Input: part model. Units: mm. Frame: model coordinates. A direction names the side the tool comes from. Coordinates: 2 decimals unless noted, no trailing zeros. Write each loop counter-clockwise with the first axis right and the second up, starting at its lowest first coordinate (ties: lowest second). Pieces come first, ordered by that corner, then holes. Notation, with made-up numbers: (44, -21) - (74, -21) arc R25 ccw to (74, -5) - close; hole circle Ø6 at (-23.5, 16.5). An arc over 180 degrees is marked (long way). Use a Markdown table: item, result. Add a question column.
Q1. Pin query (flat end, axial travel): P1, Ø1.9, axis at x = 15.5, z = 15.5, coming from the +Y side; P2, Ø2.5, axis at x = 86, z = 1, coming from the -Y side; P3, Ø7, axis at x = 2.5, z = 3, coming from the +Y side; P4, Ø2, axis at x = 9.5, z = 16.5, coming from the +Y side. Return the tip coordinate at first contact, or that it passes through.
Q2. Section query B-B (x = -85). Return the cut outline in (y, z) (3 decimals), then the cut area to 3 significant figures.
Q3. Set-up query: faces 1 (the face through (88.72, 3.94, -1.54)), 2 (the face through (93.5, 5.07, -19.72)), 3 (the face through (5.19, 6.77, 9.98)). Return all of +Z, -Z, +X, -X, +Y, -Y with unobstructed straight access to the full face (end or side cutting, diameter ignored); none if empty.
Q4. Section query A-A (x = -33.25). Return the cut outline in (y, z).
Q5. Section query C-C (z = -8). Return the cut outline in (x, y).
Q6. Section query D-D (x = 75). Return the cut outline in (y, z).
Q7. Material intervals for probe 1 along Z at (x, y) = (15.5, 4); probe 2 along Z at (x, y) = (-33.25, 4); probe 3 along X at (y, z) = (4, 15.5), sorted ascending. Write a range as from..to.
Q8. Mould query, pull axis X, two halves, no side actions, for faces 4 (the face through (-1.08, 2.79, 4.88)), 5 (the face through (-59, 10, 0)), 6 (the face through (95, 5, 0)). Classes: released by +X, released by -X, zero draft, split by the parting line, or undercut.
from build123d import *

# Parameters (mm, degrees)
SKETCH_1_W          = 190
SKETCH_1_H          = 42.3
EXTRUDE_1_DEPTH     = 10
SKETCH_2_W          = 42.5
SKETCH_2_H          = 49.677136544
CUT_EXTRUDE_1_DEPTH = 2
SKETCH_3_R          = 1.6
SKETCH_3_R_2        = 11.25
CUT_EXTRUDE_2_DEPTH = 2.5
SKETCH_4_R          = 5
CUT_EXTRUDE_3_DEPTH = 6.5
SKETCH_5_R          = 4.025
CUT_EXTRUDE_4_DEPTH = 8
SKETCH_6_R          = 1.6
CUT_EXTRUDE_5_DEPTH = 3
SKETCH_7_R          = 1.6
CUT_EXTRUDE_6_DEPTH = 3
FILLET_1_R          = 5
SKETCH_8_R          = 1.6
CUT_EXTRUDE_7_DEPTH = 9
CUT_EXTRUDE_8_REACH = 12
SKETCH_9_R          = 1.6
SKETCH_11_R         = 2.5
CUT_EXTRUDE_9_DEPTH = 11


with BuildPart() as part:
    # 草图1 → 凸台-拉伸1 (new body)
    with BuildSketch(Plane(origin=(0, 0, 0), x_dir=(1, 0, 0), z_dir=(0, 1, 0))):
        Rectangle(SKETCH_1_W, SKETCH_1_H)
    extrude(amount=EXTRUDE_1_DEPTH)

    # 草图2 → 切除-拉伸1 (cut)
    with BuildSketch(Plane(origin=(0, 10, 0), x_dir=(1, 0, 0), z_dir=(0, 1, 0))):
        Rectangle(SKETCH_2_W, SKETCH_2_H)
    extrude(amount=-CUT_EXTRUDE_1_DEPTH, mode=Mode.SUBTRACT)

    # 草图3 → 切除-拉伸2 (cut)
    with BuildSketch(Plane(origin=(0, 8, 0), x_dir=(1, 0, 0), z_dir=(0, 1, 0))):
        with Locations((-15.5, 15.5)):
            Circle(SKETCH_3_R)
        with Locations((15.5, 15.5)):
            Circle(SKETCH_3_R)
        with Locations((15.5, -15.5)):
            Circle(SKETCH_3_R)
        with Locations((-15.5, -15.5)):
            Circle(SKETCH_3_R)
        Circle(SKETCH_3_R_2)
    extrude(amount=-CUT_EXTRUDE_2_DEPTH, mode=Mode.SUBTRACT)

    # 草图4 → 切除-拉伸3 (cut, through all)
    with BuildSketch(Plane(origin=(0, 5.5, 0), x_dir=(1, 0, 0), z_dir=(0, 1, 0))):
        Circle(SKETCH_4_R)
    extrude(amount=-CUT_EXTRUDE_3_DEPTH, mode=Mode.SUBTRACT)

    # 草图5 → 切除-拉伸4 (cut)
    with BuildSketch(Plane.XZ):
        with Locations((-85, 0)):
            Circle(SKETCH_5_R)
        with Locations((85, 0)):
            Circle(SKETCH_5_R)
    extrude(amount=-CUT_EXTRUDE_4_DEPTH, mode=Mode.SUBTRACT)

    # 草图6 → 切除-拉伸5 (cut, through all)
    with BuildSketch(Plane.XZ.offset(-8)):
        with Locations((-85, 0)):
            Circle(SKETCH_6_R)
    extrude(amount=-CUT_EXTRUDE_5_DEPTH, mode=Mode.SUBTRACT)

    # 草图7 → 切除-拉伸6 (cut, through all)
    with BuildSketch(Plane.XZ.offset(-8)):
        with Locations((85, 0)):
            Circle(SKETCH_7_R)
    extrude(amount=-CUT_EXTRUDE_6_DEPTH, mode=Mode.SUBTRACT)

    # 圆角1
    fillet_1_edges = [part.edges().sort_by_distance(p)[0] for p in [
        (95, 5, 21.15),
        (-95, 5, 21.15),
        (-95, 5, -21.15),
        (95, 5, -21.15),
    ]]
    fillet(fillet_1_edges, radius=FILLET_1_R)

    # 草图8 → 切除-拉伸7 (cut, through all)
    with BuildSketch(Plane(origin=(0, 8, 0), x_dir=(1, 0, 0), z_dir=(0, 1, 0))):
        with Locations((15.5, 15.5)):
            Circle(SKETCH_8_R)
        with Locations((15.5, -15.5)):
            Circle(SKETCH_8_R)
        with Locations((-15.5, -15.5)):
            Circle(SKETCH_8_R)
        with Locations((-15.5, 15.5)):
            Circle(SKETCH_8_R)
    extrude(amount=-CUT_EXTRUDE_7_DEPTH, mode=Mode.SUBTRACT)

    # 草图9 → 切除-拉伸8 (cut, up to next)
    with BuildSketch(Plane(origin=(0, 10, 0), x_dir=(1, 0, 0), z_dir=(0, 1, 0)), mode=Mode.PRIVATE) as cut_extrude_8_sk1:
        with Locations((-33.25, -13.15)):
            Circle(SKETCH_9_R)
    cut_extrude_8_tool1 = extrude(cut_extrude_8_sk1.sketch, amount=-CUT_EXTRUDE_8_REACH, mode=Mode.PRIVATE) & part.part
    add(cut_extrude_8_tool1.solids().sort_by_distance((-33.25, 10, 13.15))[0], mode=Mode.SUBTRACT)

    # 草图11 → 切除-拉伸9 (cut, through all)
    with BuildSketch(Plane(origin=(0, 10, 0), x_dir=(1, 0, 0), z_dir=(0, 1, 0))):
        with Locations((75, 16.15)):
            Circle(SKETCH_11_R)
    extrude(amount=-CUT_EXTRUDE_9_DEPTH, mode=Mode.SUBTRACT)


solid = part.part
Values follow:
| question | item | result |
|---|---|---|
| 1 | P1 | through |
| 1 | P2 | y = 8 |
| 1 | P3 | y = 5.5 |
| 1 | P4 | y = 8 |
| 2 | outline | (0, -21.15) - (10, -21.15) - (10, -1.6) - (8, -1.6) - (8, -4.025) - (0, -4.025) - close; (0, 4.025) - (8, 4.025) - (8, 1.6) - (10, 1.6) - (10, 21.15) - (0, 21.15) - close |
| 2 | area | 352 mm2 |
| 3 | face 1 | -Y |
| 3 | face 2 | -Z, +X, +Y, -Y |
| 3 | face 3 | +Y |
| 4 | outline | (0, -21.15) - (10, -21.15) - (10, 11.55) - (0, 11.55) - close; (0, 14.75) - (10, 14.75) - (10, 21.15) - (0, 21.15) - close |
| 5 | outline | (-95, 0) - (95, 0) - (95, 10) - (21.25, 10) - (21.25, 8) - (7.91, 8) - (7.91, 5.5) - (-7.91, 5.5) - (-7.91, 8) - (-21.25, 8) - (-21.25, 10) - (-95, 10) - close |
| 6 | outline | (0, -21.15) - (10, -21.15) - (10, -18.65) - (0, -18.65) - close; (0, -13.65) - (10, -13.65) - (10, 21.15) - (0, 21.15) - close |
| 7 | probe 1 | -21.15..-17.1, -13.9..13.9, 17.1..21.15 |
| 7 | probe 2 | -21.15..11.55, 14.75..21.15 |
| 7 | probe 3 | -95..-17.1, -13.9..13.9, 17.1..95 |
| 8 | face 4 | undercut |
| 8 | face 5 | zero draft |
| 8 | face 6 | released by +X |
